Could you check a few things on this model? Use its own coordinates, in mm. A direction names the side the tool comes from. Coordinates: 2 decimals unless noted, no trailing zeros. Order: outer loops, then holes, each group sorted by start corner. A loop starts at its lowest first (then second) coordinate and runs counter-clockwise, first axis right, second up. Notation, with made-up numbers: (-0.5, -9.5) -> (20.5, -9.5) arc R18 ccw to (20.5, 8.5) -> close; hole circle Ø6 at (30.5, 76.25). An arc over 180 degrees is marked (long way). Use a Markdown table: item, result. Add a question column.
1) Thinking about a two-plate mould opening in X: for faces 1 (the flat face through (14.85, -24, 7.96)), 2 (the flat face through (14.76, -26.54, 6.91)), 3 (the flat face through (11.6, 19.2, 11.25)), which applies, +X half, -X half, draft (parallel to the pull), parting line (faces both ways), or undercut?
2) Which directions (+Z, -Z, +X, -X, +Y, -Y) give clear straight access to the entire face, cutting with the end or side of a thin tool? Please do faces 4 (the flat face through (8.882, 20, 6)), 5 (the cylindrical face through (17.87, 25.38, 6.54)), 6 (the flat face through (19, 29.94, 7)).
3) If we section it at B-B (x = 10.16): Give the number of separate pieces and of enclosed holes in the cut face, plus the area to 3 significant figures.
4) If I drill on L1, parallel to Y at x = 10.16, z = 6.5; L2, parallel to Y at x = -10, z = 0.85; L3, parallel to X at y = -1, z = 5.5, over which ranges is the centre line in solid material (lowest first)? Write a range as [from, to].
5) If we section it at A-A (y = -26.5): Write out the boundary of the cut face in (x, z).
6) Will these pins go through, and if not, where does the flat tip stop? pin 1 Ø4 at (x, z) = (-13.5, 3.5) entering from -Y; pin 2 Ø1.1 at (y, z) = (-31, 3.5) entering from +X; pin 3 Ø0.6 at (y, z) = (33.5, 5.5) entering from -X; pin 4 Ø2.5 at (x, y) = (19.25, 24.94) entering from +Z.
```python
from build123d import *

# Parameters (mm, degrees)
SKETCH1_W                 = 28
SKETCH1_H                 = 68
BOSS_EXTRUDE1_DEPTH       = 1.25
SKETCH21_W                = 1.925
SKETCH21_H                = 1
BOSS_EXTRUDE10_DEPTH      = 3
SKETCH22_W                = 2.89
SKETCH22_H                = 3
SKETCH22_R                = 1.25
BOSS_EXTRUDE11_DEPTH      = 10
SKETCH7_W                 = 28
SKETCH7_H                 = 68
SKETCH7_W_2               = 25.5
SKETCH7_H_2               = 65.5
BOSS_EXTRUDE4_DEPTH       = 7.75
SKETCH18_W                = 13
SKETCH18_H                = 4
CUT_EXTRUDE10_DEPTH       = 1.25
SKETCH13_R                = 1.05
BOSS_EXTRUDE7_DEPTH       = 5
LPATTERN2_COUNT           = 4
LPATTERN2_PITCH           = 5
SKETCH14_W                = 10
SKETCH14_H                = 5
CUT_EXTRUDE5_DEPTH        = 5
FILLET1_R                 = 1
FILLET7_R                 = 1
M4_CLEARANCE_HOLE1_D      = 4.8
SKETCH26_R                = 1.45
BOSS_EXTRUDE12_DEPTH      = 5
FILLET10_R                = 1
FILLET12_R                = 1
BOSS_EXTRUDE13_DEPTH      = 5
BOSS_EXTRUDE13_DEPTH_BACK = 20
SKETCH28_R                = 1.05
CUT_EXTRUDE11_DEPTH       = 44.250722537
CUT_EXTRUDE11_DEPTH_BACK  = 44.250722537
SKETCH29_R                = 1.25


with BuildPart() as part:
    # Sketch1 → Boss-Extrude1 (new body)
    with BuildSketch(Plane.XY):
        Rectangle(SKETCH1_W, SKETCH1_H)
    extrude(amount=BOSS_EXTRUDE1_DEPTH)

    # Sketch21 → Boss-Extrude10 (add)
    with BuildSketch(Plane.XY.offset(1.25)):
        with Locations((-8.365871065, 31)):
            Rectangle(SKETCH21_W, SKETCH21_H)
        with Locations((7.559128935, 31)):
            Rectangle(SKETCH21_W, SKETCH21_H)
        with Locations((7.559128935, -30.993333443)):
            Rectangle(SKETCH21_W, SKETCH21_H)
        with Locations((-8.365871065, -30.993333443)):
            Rectangle(SKETCH21_W, SKETCH21_H)
    extrude(amount=BOSS_EXTRUDE10_DEPTH)

    # Sketch22 → Boss-Extrude11 (add)
    # profile 1 of 4: a face of its own
    with BuildSketch(Plane.XY.offset(1.25)):
        with Locations((10.326628935, 19.170761532)):
            Rectangle(SKETCH22_W, SKETCH22_H)
        with Locations((10.16, 19.170761532)):
            Circle(SKETCH22_R, mode=Mode.SUBTRACT)
    # profile 2 of 4: a face of its own
    with BuildSketch(Plane.XY.offset(1.25)):
        with Locations((-10.326628935, 19.170761532)):
            Rectangle(SKETCH22_W, SKETCH22_H)
        with Locations(Location((-10.16, 19.170761532, 0), (0, 0, 180))):
            Circle(SKETCH22_R, mode=Mode.SUBTRACT)
    # profile 3 of 4: a face of its own
    with BuildSketch(Plane.XY.offset(1.25)):
        with Locations((10.326628935, 6.470761532)):
            Rectangle(SKETCH22_W, SKETCH22_H)
        with Locations(Location((10.16, 6.470761532, 0), (0, 0, 180))):
            Circle(SKETCH22_R, mode=Mode.SUBTRACT)
    # profile 4 of 4: a face of its own
    with BuildSketch(Plane.XY.offset(1.25)):
        with Locations((-10.326628935, 6.470761532)):
            Rectangle(SKETCH22_W, SKETCH22_H)
        with Locations((-10.16, 6.470761532)):
            Circle(SKETCH22_R, mode=Mode.SUBTRACT)
    extrude(amount=BOSS_EXTRUDE11_DEPTH)

    # Sketch7 → Boss-Extrude4 (add)
    with BuildSketch(Plane.XY.offset(1.25)):
        Rectangle(SKETCH7_W, SKETCH7_H)
        Rectangle(SKETCH7_W_2, SKETCH7_H_2, mode=Mode.SUBTRACT)
    extrude(amount=BOSS_EXTRUDE4_DEPTH)

    # Sketch18 → Cut-Extrude10 (cut)
    with BuildSketch(Plane(origin=(0, 34, 0), x_dir=(1, 0, 0), z_dir=(0, 1, 0))):
        with Locations((0, -5.15)):
            Rectangle(SKETCH18_W, SKETCH18_H)
    extrude(amount=-CUT_EXTRUDE10_DEPTH, mode=Mode.SUBTRACT)

    # Sketch13 → Boss-Extrude7 (add)
    with BuildSketch(Plane.XZ.offset(34)):
        with BuildLine():
            Line((15.5, 7.5), (14, 6.303164343))
            Line((14, 6.303164343), (14, 9))
            ThreePointArc((14, 9), (16.560660172, 10.060660172), (15.5, 7.5))
        make_face()
        with Locations(Location((15.5, 9, 0), (0, 0, 270))):
            Circle(SKETCH13_R, mode=Mode.SUBTRACT)
    boss_extrude7 = extrude(amount=-BOSS_EXTRUDE7_DEPTH)

    # LPattern2: Boss-Extrude7 ×4, 1 skipped
    with Locations(*[(0, i * LPATTERN2_PITCH, 0) for i in range(1, LPATTERN2_COUNT) if i not in (2,)]):
        add(boss_extrude7)

    # Sketch14 → Cut-Extrude5 (cut)
    with BuildSketch(Plane(origin=(14, 0, 0), x_dir=(0, 0, -1), z_dir=(1, 0, 0))):
        with Locations((-6.85234732, -31.5)):
            Rectangle(SKETCH14_W, SKETCH14_H)
    extrude(amount=CUT_EXTRUDE5_DEPTH, mode=Mode.SUBTRACT)

    # Fillet1
    fillet1_edges = [part.edges().sort_by_distance(p)[0] for p in [
        (14, -34, 4.5),
        (0, 34, 0),
        (14, 0, 0),
        (0, -34, 0),
        (-14, 0, 0),
        (-14, 34, 4.5),
        (14, 34, 4.5),
        (-14, -34, 4.5),
    ]]
    fillet(fillet1_edges, radius=FILLET1_R)

    # Fillet7
    fillet7_edges = [part.edges().sort_by_distance(p)[0] for p in [
        (-6.5, 33.375, 3.15),
        (-6.5, 33.375, 7.15),
        (6.5, 33.375, 7.15),
        (6.5, 33.375, 3.15),
    ]]
    fillet(fillet7_edges, radius=FILLET7_R)

    # M4 Clearance Hole1 (through all)
    with Locations(Plane.XY.offset(1.25)):
        with Locations((-10, 26.525248178), (10, 26.525248178), (10, -8.474751822), (-10, -8.474751822)):
            Hole(M4_CLEARANCE_HOLE1_D / 2)

    # Sketch26 → Boss-Extrude12 (add)
    with BuildSketch(Plane.XY.offset(9)):
        Polygon((-14, 29.939793189), (-24.25, 29.939793189), (-24.25, -8.060206811), (-14, -8.060206811), (-14, -3.060206811), (-20.799999976, -3.060206811), (-21.025, 19.939793189), (-14, 19.939793189), align=None)
        with Locations((-19.25, 24.941355933)):
            Circle(SKETCH26_R, mode=Mode.SUBTRACT)
    boss_extrude12 = extrude(amount=-BOSS_EXTRUDE12_DEPTH)

    # Fillet10
    fillet10_edges = [part.edges().sort_by_distance(p)[0] for p in [
        (-14, 29.939793189, 6.5),
        (-14, 19.939793189, 6.5),
        (-21.025, 19.939793189, 6.5),
        (-20.799999976, -3.060206811, 6.5),
        (-14, -3.060206811, 6.5),
        (-14, -8.060206811, 6.5),
        (-24.25, -8.060206811, 6.5),
        (-24.25, 29.939793189, 6.5),
    ]]
    fillet(fillet10_edges, radius=FILLET10_R)

    # Mirror2: Boss-Extrude12 across plane
    add(boss_extrude12.mirror(Plane.ZY))

    # Fillet12
    fillet12_edges = [part.edges().sort_by_distance(p)[0] for p in [
        (14, 19.939793189, 6.5),
        (14, 29.939793189, 6.5),
        (24.25, 29.939793189, 6.5),
        (24.25, -8.060206811, 6.5),
        (14, -8.060206811, 6.5),
        (14, -3.060206811, 6.5),
        (20.799999976, -3.060206811, 6.5),
        (21.025, 19.939793189, 6.5),
    ]]
    fillet(fillet12_edges, radius=FILLET12_R)

    # Sketch28 → Boss-Extrude13 (add, two sides: drawn at the far end of the back side and taken through both)
    with BuildSketch(Plane(origin=(0, -29, 0), x_dir=(-1, 0, 0), z_dir=(0, -1, 0)).offset(-BOSS_EXTRUDE13_DEPTH_BACK)):
        with Locations(Location((-15.5, -9, 0), (0, 0, 180))):
            Circle(SKETCH28_R)
    extrude(amount=BOSS_EXTRUDE13_DEPTH + BOSS_EXTRUDE13_DEPTH_BACK)

    # Sketch29 → Cut-Extrude11 (cut, two sides: drawn at the far end of the back side and taken through both)
    with BuildSketch(Plane.XY.offset(11.25).offset(-CUT_EXTRUDE11_DEPTH_BACK)):
        with Locations(Location((-10.16, 19.170761532, 0), (0, 0, 180))):
            Circle(SKETCH29_R)
        with Locations((-10.16, 6.470761532)):
            Circle(SKETCH29_R)
        with Locations(Location((10.16, 6.470761532, 0), (0, 0, 180))):
            Circle(SKETCH29_R)
        with Locations((10.16, 19.170761532)):
            Circle(SKETCH29_R)
    extrude(amount=CUT_EXTRUDE11_DEPTH + CUT_EXTRUDE11_DEPTH_BACK, mode=Mode.SUBTRACT)


solid = part.part
```
Answer sheet:
| question | item | result |
|---|---|---|
| 1 | face 1 | undercut |
| 1 | face 2 | +X half |
| 1 | face 3 | draft |
| 2 | face 4 | +Z |
| 2 | face 5 | +Z, -Z |
| 2 | face 6 | +Z, -Z, +X, +Y |
| 3 | separate pieces | 5 |
| 3 | enclosed holes | 0 |
| 3 | area | 95.7 mm2 |
| 4 | L1 | [-34, -32.75], [4.97, 5.22], [7.72, 7.97], [17.67, 17.92], [20.42, 20.67], [32.75, 34] |
| 4 | L2 | [-33.99, -10.87], [-6.07, 5.23], [7.71, 17.93], [20.41, 24.13], [28.93, 33.99] |
| 4 | L3 | [-24.25, -20.82], [-14, -12.75], [12.75, 14], [20.82, 24.25] |
| 5 | outline | (-14, 1) arc R1 ccw to (-13, 0) -> (13, 0) arc R1 ccw to (14, 1) -> (14, 6.3) -> (15.5, 7.5) arc R1.5 ccw (long way) to (14, 9) -> (12.75, 9) -> (12.75, 1.25) -> (-12.75, 1.25) -> (-12.75, 9) -> (-14, 9) -> close |
| 6 | pin 1 | y = -34 |
| 6 | pin 2 | x = 14 |
| 6 | pin 3 | x = -13.98 |
| 6 | pin 4 | through |
